Geometry check sheet. Reference: drawing and pictorial views, mm from the part's lowest x, y, z. Give positions to 0.01 mm unless a question says otherwise; leave off trailing zeros. Order: outer loops, then holes, each group sorted by start corner. A loop starts at its lowest first (then second) coordinate and runs counter-clockwise, first axis right, second up. Notation, with made-up numbers: (-32, 29.5) -> (-24, 29.5) arc R21 cw to (-24, 68.5) -> close; hole circle Ø4 at (13.25, -26). An arc over 180 degrees is marked (long way). Write each question's results on one line, items separated by ' | '.
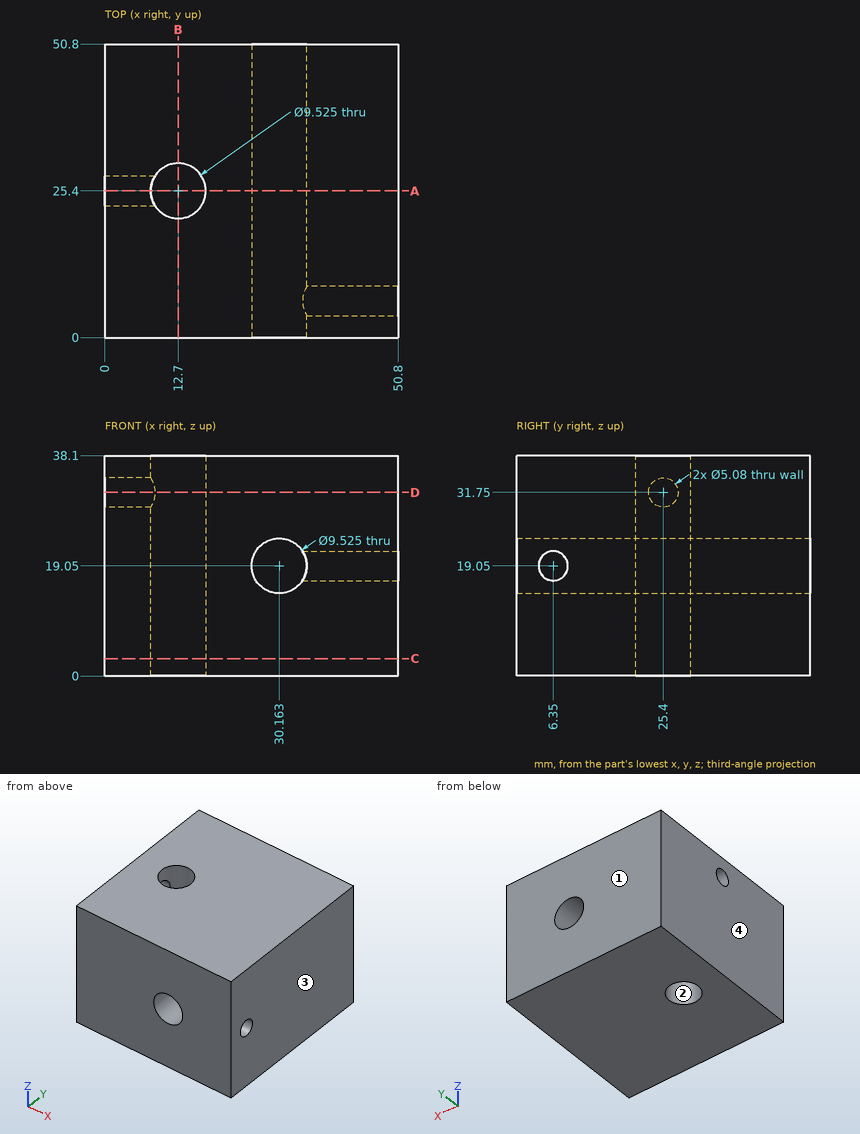
1. Gauge pin test, flat end, axial feed: pin 1 Ø3 at (y, z) = (6.35, 19.05) entering from +X. Record the tip position at first contact, or that the pin passes through.
Verdict:
pin 1: stops at x = 25.64
2. Section check D-D on z = 31.75. Record the cut outline in (x, y) (1 decimal), then the cut area to 3 significant figures.
Verdict:
outline: (0, 0) -> (50.8, 0) -> (50.8, 50.8) -> (0, 50.8) -> (0, 27.9) -> (8.7, 27.9) arc R4.8 cw (long way) to (8.7, 22.9) -> (0, 22.9) -> close | area: 2,470 mm^2
3. Material ranges on probe 1 along Y at (x, z) = (13, 8); probe 2 along X at (y, z) = (25, 13) (1 decimal); probe 3 along Z at (x, y) = (32.5, 29), recorded low to high. Write a range as from..to.
Verdict:
probe 1: y = 0..20.65, 30.15..50.8 | probe 2: x = 0..8, 17.4..50.8 | probe 3: z = 0..14.9, 23.2..38.1
4. Section check A-A on y = 25.4. Give the number of separate pieces and of enclosed holes in the cut face, then the cut area to 3 significant figures.
Verdict:
separate pieces: 3 | enclosed holes: 1 | area: 1,460 mm^2
5. Section check B-B on x = 12.7. Record the cut outline in (y, z), then the cut area to 3 significant figures.
Verdict:
outline: (0, 0) -> (20.64, 0) -> (20.64, 38.1) -> (0, 38.1) -> close; (30.16, 0) -> (50.8, 0) -> (50.8, 38.1) -> (30.16, 38.1) -> close | area: 1,570 mm^2
6. Section check C-C on z = 3. Record the cut outline in (x, y) (1 decimal), then the cut area to 3 significant figures.
Verdict:
outline: (0, 0) -> (50.8, 0) -> (50.8, 50.8) -> (0, 50.8) -> close; hole circle Ø9.5 at (12.7, 25.4) | area: 2,510 mm^2
7. Mould release check, pull along X, two halves, no side actions. Record for the marked faces 1, 2, 3 and 4: +X half, -X half, draft (parallel to the pull), parting line (faces both ways), or undercut.
Verdict:
face 1: draft | face 2: undercut | face 3: +X half | face 4: -X half
